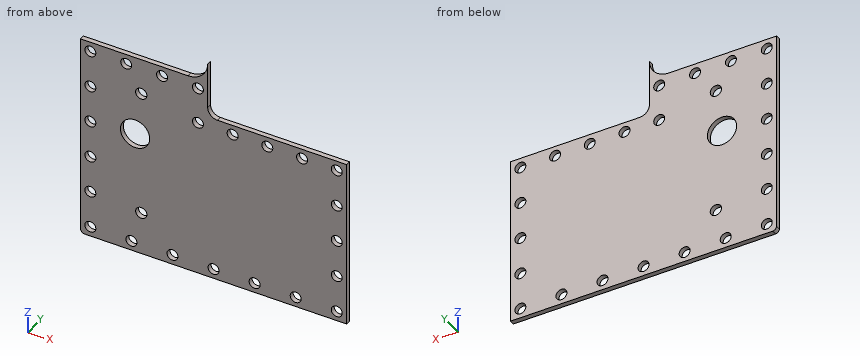
from build123d import *

# Parameters (mm, degrees)
BOSS_EXTRUDE1_DEPTH     = 1.5875
FILLET1_R               = 3.175
SKETCH2_R               = 4.750027573
SKETCH2_R_2             = 1.830008083
CUT_EXTRUDE1_DEPTH      = 1
CUT_EXTRUDE1_DEPTH_BACK = 2.5875
SKETCH3_R               = 1.778
CUT_EXTRUDE2_DEPTH      = 1
CUT_EXTRUDE2_DEPTH_BACK = 2.5875


with BuildPart() as part:
    # Sketch1 → Boss-Extrude1 (new body)
    with BuildSketch(Plane(origin=(0, 0, 0), x_dir=(1, 0, 0), z_dir=(0, 1, 0))):
        with BuildLine():
            Line((-8.89, -66.675), (-43.815, -66.675))
            Line((-43.815, -66.675), (-43.815, -1.27))
            ThreePointArc((-43.815, -1.27), (-43.443025612, -0.371974388), (-42.545, 0))
            Line((-42.545, 0), (42.545, 0))
            Line((42.545, 0), (42.545, -54.843091388))
            Line((42.545, -54.843091388), (-2.54, -54.843091388))
            Line((-2.54, -54.843091388), (-2.54, -73.025))
            ThreePointArc((-2.54, -73.025), (-4.399871939, -68.534871939), (-8.89, -66.675))
        make_face()
    extrude(amount=BOSS_EXTRUDE1_DEPTH)

    # Fillet1
    fillet1_edges = [part.edges().sort_by_distance(p)[0] for p in [
        (-2.54, 0.79375, 54.843091388),
    ]]
    fillet(fillet1_edges, radius=FILLET1_R)

    # Sketch2 → Cut-Extrude1 (cut, two sides)
    with BuildSketch(Plane(origin=(0, 1.5875, 0), x_dir=(-1, 0, 0), z_dir=(0, 1, 0))) as cut_extrude1_sk:
        with Locations((26.115028378, 40.470331632)):
            Circle(SKETCH2_R)
        with Locations((24.115016768, 54.970415803)):
            Circle(SKETCH2_R_2)
        with Locations((24.114889767, 13.97)):
            Circle(SKETCH2_R_2)
    extrude(amount=CUT_EXTRUDE1_DEPTH, mode=Mode.SUBTRACT)
    extrude(cut_extrude1_sk.sketch, amount=-CUT_EXTRUDE1_DEPTH_BACK, mode=Mode.SUBTRACT)

    # Sketch3 → Cut-Extrude2 (cut, two sides)
    with BuildSketch(Plane(origin=(0, 1.5875, 0), x_dir=(-1, 0, 0), z_dir=(0, 1, 0))) as cut_extrude2_sk:
        with Locations((27.305, 3.175)):
            Circle(SKETCH3_R)
        with Locations((13.97, 3.175)):
            Circle(SKETCH3_R)
        with Locations((0.635, 3.175)):
            Circle(SKETCH3_R)
        with Locations((-12.7, 3.175)):
            Circle(SKETCH3_R)
        with Locations((-26.035, 3.175)):
            Circle(SKETCH3_R)
        with Locations((-39.37, 3.175)):
            Circle(SKETCH3_R)
        with Locations((-39.37, 15.298272847)):
            Circle(SKETCH3_R)
        with Locations((-39.37, 27.421545694)):
            Circle(SKETCH3_R)
        with Locations((-39.37, 39.544818541)):
            Circle(SKETCH3_R)
        with Locations((-39.37, 51.668091388)):
            Circle(SKETCH3_R)
        with Locations((-28.09875, 51.668091388)):
            Circle(SKETCH3_R)
        with Locations((-16.8275, 51.668091388)):
            Circle(SKETCH3_R)
        with Locations((-5.55625, 51.668091388)):
            Circle(SKETCH3_R)
        with Locations((5.715, 51.668091388)):
            Circle(SKETCH3_R)
        with Locations((5.715, 63.5)):
            Circle(SKETCH3_R)
        with Locations((17.356666667, 63.5)):
            Circle(SKETCH3_R)
        with Locations((28.998333333, 63.5)):
            Circle(SKETCH3_R)
        with Locations((40.64, 63.5)):
            Circle(SKETCH3_R)
        with Locations((40.64, 51.435)):
            Circle(SKETCH3_R)
        with Locations((40.64, 39.37)):
            Circle(SKETCH3_R)
        with Locations((40.64, 27.305)):
            Circle(SKETCH3_R)
        with Locations((40.64, 15.24)):
            Circle(SKETCH3_R)
        with Locations((40.64, 3.175)):
            Circle(SKETCH3_R)
    extrude(amount=CUT_EXTRUDE2_DEPTH, mode=Mode.SUBTRACT)
    extrude(cut_extrude2_sk.sketch, amount=-CUT_EXTRUDE2_DEPTH_BACK, mode=Mode.SUBTRACT)


solid = part.part
Could you check a few things on this model? Use its own coordinates, in mm. Give positions to 0.01 mm unless a question says otherwise; leave off trailing zeros. Order: outer loops, then holes, each group sorted by start corner. A loop starts at its lowest first (then second) coordinate and runs counter-clockwise, first axis right, second up.
Item 1: If we section it at D-D, the plane x = -17.5: Write out the boundary of the cut face in (y, z) (1 decimal).
Item 2: I need wall thicknesses on line 1 (X direction, y = 0.85, z = 27.5) (3 decimals); line 2 (Z direction, x = 39.37, y = 1.05); line 3 (Z direction, x = 17, y = 0.95). Which ranges of each line are inside material? Lowest first, please.
Item 3: I'm going to push a flat-ended pin straight in: pin 1 (4.5 mm diameter, centred on x = -5.715, z = 63.5, fed in from -Y). Where does the tip first touch, or does it pass through?
Item 4: If we section it at C-C, the plane x = 12.7: Write out the boundary of the cut face in (y, z), plus the area to 3 significant figures.
Item 5: If we section it at A-A, the plane x = 39.37: Write out the boundary of the cut face in (y, z).
Item 6: If we section it at B-B, the plane z = 63.5: Write out the boundary of the cut face in (x, y) (1 decimal), plus the area to 3 significant figures.
Values:
1. outline: (0, 0) - (1.6, 0) - (1.6, 61.7) - (0, 61.7) - close; (0, 65.3) - (1.6, 65.3) - (1.6, 66.7) - (0, 66.7) - close
2. line 1: x = -43.815 to -42.407, -38.873 to 37.594, 41.146 to 42.545
2. line 2: z = 0 to 1.4, 4.95 to 13.52, 17.08 to 25.64, 29.2 to 37.77, 41.32 to 49.89, 53.45 to 54.84
2. line 3: z = 0 to 49.9, 53.44 to 54.84
3. pin 1: stops at y = 0
4. outline: (0, 0) - (1.59, 0) - (1.59, 1.4) - (0, 1.4) - close; (0, 4.95) - (1.59, 4.95) - (1.59, 54.84) - (0, 54.84) - close
4. area: 81.4 mm2
5. outline: (0, 0) - (1.59, 0) - (1.59, 1.4) - (0, 1.4) - close; (0, 4.95) - (1.59, 4.95) - (1.59, 13.52) - (0, 13.52) - close; (0, 17.08) - (1.59, 17.08) - (1.59, 25.64) - (0, 25.64) - close; (0, 29.2) - (1.59, 29.2) - (1.59, 37.77) - (0, 37.77) - close; (0, 41.32) - (1.59, 41.32) - (1.59, 49.89) - (0, 49.89) - close; (0, 53.45) - (1.59, 53.45) - (1.59, 54.84) - (0, 54.84) - close
6. outline: (-43.8, 0) - (-42.4, 0) - (-42.4, 1.6) - (-43.8, 1.6) - close; (-38.9, 0) - (-30.8, 0) - (-30.8, 1.6) - (-38.9, 1.6) - close; (-27.2, 0) - (-19.1, 0) - (-19.1, 1.6) - (-27.2, 1.6) - close; (-15.6, 0) - (-7.5, 0) - (-7.5, 1.6) - (-15.6, 1.6) - close; (-3.9, 0) - (-2.5, 0) - (-2.5, 1.6) - (-3.9, 1.6) - close
6. area: 42.9 mm2
